Print and shaded views of the part. All mm, measured from the part's lowest x, y and z. A direction names the side the tool comes from. Give positions to 0.01 mm unless a question says otherwise; leave off trailing zeros. Loops run counter-clockwise (first coordinate to the right, second up) from the corner with the lowest first, then second, coordinate; pieces in that order, holes last. Notation, with made-up numbers: (86, -25) -> (104, -25) arc R26 ccw to (104, 2) -> close; hole circle Ø9 at (-39.5, 11). An arc over 180 degrees is marked (long way). Write each question's results on one line, items separated by ' | '. Start each with the question number.
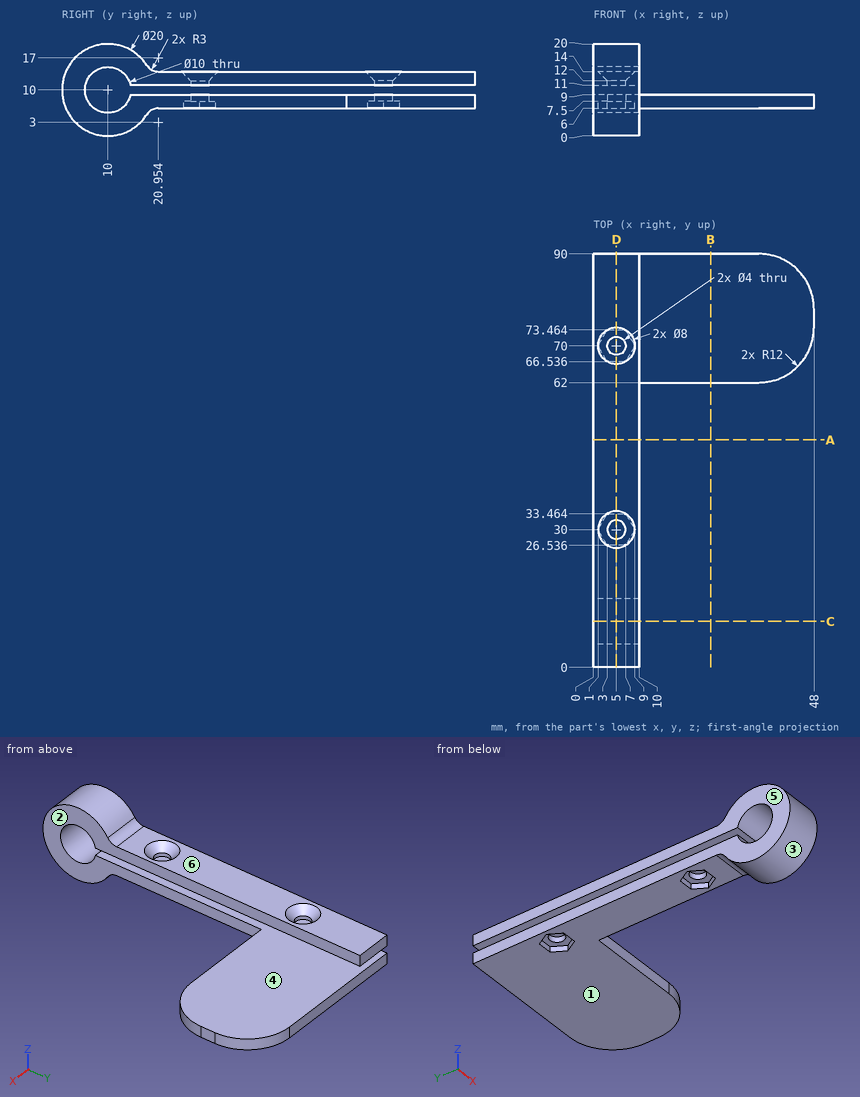
Q1. Saw through at A-A, the plane y = 49.5. List the corners of the cut face in (x, z).
Q2. Saw through at B-B, the plane x = 25.5. List the corners of the cut face in (y, z).
Q3. Saw through at D-D, the plane x = 5. Give the number of separate pieces and of enclosed holes in the cut face, then the cut area to 3 significant figures.
Q4. Wall check: L1, parallel to Z at x = 7.5, y = 37; L2, parallel to X at y = 30, z = 11.4; L3, parallel to X at y = 11.5, z = 1.75. Give the ranges that are in metal, low to high.
Q5. Drop flat-ended pins along their axis: pin 1 (6.5 mm diameter, centred on x = 5, y = 30, fed in from -Z); pin 2 (11 mm diameter, centred on x = 4, y = 48.5, fed in from +Z); pin 3 (12 mm diameter, centred on y = 27, z = 13.5, fed in from +X). Give the stop position or say it passes through.
Q6. Mould opens along Z. For the marked faces 4, 5 and 6 say: pulls with the +Z half, pulls with the -Z half, needs draft (parallel to the pull), parting line crosses it, or undercut.
Q7. Which spindle directions (+Z, -Z, +X, -X, +Y, -Y) get a long thin tool onto all of the face, cutting with end or side? Do the marked faces 1, 2 and 3. Say none if no direction does.
Q8. Saw through at C-C, the plane y = 10. List the corners of the cut face in (x, z), then the cut area to 3 significant figures.
Answer block:
1) outline: (0, 6) -> (10, 6) -> (10, 9) -> (0, 9) -> close; (0, 11) -> (10, 11) -> (10, 14) -> (0, 14) -> close
2) outline: (62, 6) -> (90, 6) -> (90, 9) -> (62, 9) -> close
3) separate pieces: 5 | enclosed holes: 0 | area: 584 mm2
4) L1: z = 6 to 9, 11 to 14 | L2: x = 0 to 3, 7 to 10 | L3: x = 0 to 10
5) pin 1: stops at z = 7.5 | pin 2: stops at z = 14 | pin 3: stops at x = 10
6) face 4: undercut | face 5: needs draft | face 6: pulls with the +Z half
7) face 1: -Z, +X, -X, +Y | face 2: +Z, +X, -Y | face 3: +X, -X
8) outline: (0, 0) -> (10, 0) -> (10, 5) -> (0, 5) -> close; (0, 15) -> (10, 15) -> (10, 20) -> (0, 20) -> close | area: 100 mm2
